Geometry: final body of the model. Coordinates: model frame, mm. A direction names the side the tool comes from. Coordinates: 2 decimals unless noted, no trailing zeros. Order: outer loops, then holes, each group sorted by start corner. A loop starts at its lowest first (then second) coordinate and runs counter-clockwise, first axis right, second up. Notation, with made-up numbers: (33.5, 85.5) - (87.5, 85.5) arc R20 cw to (87.5, 120.5) - close; hole circle Ø4 at (-2, 71.25). An arc over 180 degrees is marked (long way). Use one line per item in the form item = value. Start each with the question number.
```python
from build123d import *

# Parameters (mm, degrees)
CROQUIS1_R              = 1
CROQUIS1_R_2            = 1.25
SALIENTE_EXTRUIR1_DEPTH = 3
CORTAR_EXTRUIR1_DEPTH   = 1.5
CROQUIS3_R              = 2.1
CORTAR_EXTRUIR2_DEPTH   = 0.75
CROQUIS4_R              = 0.5
CORTAR_EXTRUIR3_DEPTH   = 23.410934831
CHAFL_N1_SIZE           = 0.5


with BuildPart() as part:
    # Croquis1 → Saliente-Extruir1 (new body)
    with BuildSketch(Plane.XY):
        with BuildLine():
            Line((0.210526316, 3.994455992), (19.157894737, 2.995841994))
            ThreePointArc((19.157894737, 2.995841994), (22, 0), (19.157894737, -2.995841994))
            Line((19.157894737, -2.995841994), (0.210526316, -3.994455992))
            ThreePointArc((0.210526316, -3.994455992), (-4, 0), (0.210526316, 3.994455992))
        make_face()
        Circle(CROQUIS1_R, mode=Mode.SUBTRACT)
        with Locations((19, 0)):
            Circle(CROQUIS1_R_2, mode=Mode.SUBTRACT)
    extrude(amount=SALIENTE_EXTRUIR1_DEPTH)

    # Croquis2 → Cortar-Extruir1 (cut)
    with BuildSketch(Plane(origin=(0, 0, 0), x_dir=(-1, 0, 0), z_dir=(0, 0, -1))):
        with BuildLine():
            Line((-15.154651163, 2.247564934), (-0.137209302, 2.946807358))
            ThreePointArc((-0.137209302, 2.946807358), (2.95, 0), (-0.137209302, -2.946807358))
            Line((-0.137209302, -2.946807358), (-15.154651163, -2.247564934))
            ThreePointArc((-15.154651163, -2.247564934), (-17.3, 0), (-15.154651163, 2.247564934))
        make_face()
    extrude(amount=-CORTAR_EXTRUIR1_DEPTH, mode=Mode.SUBTRACT)

    # Croquis3 → Cortar-Extruir2 (cut)
    with BuildSketch(Plane(origin=(0, 0, 1.5), x_dir=(-1, 0, 0), z_dir=(0, 0, -1))):
        Circle(CROQUIS3_R)
    extrude(amount=-CORTAR_EXTRUIR2_DEPTH, mode=Mode.SUBTRACT)

    # Croquis4 → Cortar-Extruir3 (cut, through all)
    with BuildSketch(Plane(origin=(0, 0, 1.5), x_dir=(-1, 0, 0), z_dir=(0, 0, -1))):
        with Locations((-15.05, 0)):
            Circle(CROQUIS4_R)
    extrude(amount=-CORTAR_EXTRUIR3_DEPTH, mode=Mode.SUBTRACT)

    # Chaflán1
    chafl_n1_edges = [part.edges().sort_by_distance(p)[0] for p in [
        (22, 0, 3),
        (9.684210526, 3.495148993, 3),
        (-4, 0, 3),
        (9.684210526, -3.495148993, 3),
    ]]
    chamfer(chafl_n1_edges, length=CHAFL_N1_SIZE)


solid = part.part
```
(1) Set-up query: faces 1 (the flat face through (7.751, 2.592, 0.74)), 2 (the cylindrical face through (22, 0, 1)). Return all of +Z, -Z, +X, -X, +Y, -Y with unobstructed straight access to the full face (end or side cutting, diameter ignored); none if empty.
(2) Cut plane A-A on y = 0. Return the cut outline in (x, z).
(3) Draft query along X for faces 3 (the cylindrical face through (14.573, 0.15, 2.24)), 4 (the flat face through (9.817, -3.488, 1.232)), 5 (the flat face through (9, 0, 3)). Return one class per face: released by +X, released by -X, zero draft, split by the parting line, or undercut.
(4) Contact query for flat-ended pins moving along their axis: pin 1 Ø2 at (x, y) = (19, 0) entering from +Z; pin 2 Ø1.5 at (x, y) = (10.5, -0.5) entering from -Z. Output: stop coordinate, or through.
(5) Cut plane C-C on x = 11.5. Return the cut outline in (y, z), plus the area to 3 significant figures.
(6) Material intervals for L1, parallel to X at y = -0.5, z = 0.7; L2, parallel to Z at x = 16, y = -0.25; L3, parallel to X at y = -1, z = 2.2, sorted ascending. Write a range as from..to.
(7) Cut plane D-D on x = 8.25. Return the cut outline in (y, z), plus the area to 3 significant figures.
Check sheet entries:
q1.face_1 = -Z
q1.face_2 = +Z, -Z, +X
q2.outline = (-4, 0) - (-2.95, 0) - (-2.95, 1.5) - (-2.1, 1.5) - (-2.1, 2.25) - (-1, 2.25) - (-1, 3) - (-3.5, 3) - (-4, 2.5) - close; (1, 2.25) - (2.1, 2.25) - (2.1, 1.5) - (14.55, 1.5) - (14.55, 3) - (1, 3) - close; (15.55, 1.5) - (17.3, 1.5) - (17.3, 0) - (17.75, 0) - (17.75, 3) - (15.55, 3) - close; (20.25, 0) - (22, 0) - (22, 2.5) - (21.5, 3) - (20.25, 3) - close
q3.face_3 = undercut
q3.face_4 = released by +X
q3.face_5 = zero draft
q4.pin_1 = through
q4.pin_2 = 1.5
q5.outline = (-3.4, 0) - (-2.42, 0) - (-2.42, 1.5) - (2.42, 1.5) - (2.42, 0) - (3.4, 0) - (3.4, 2.5) - (2.9, 3) - (-2.9, 3) - (-3.4, 2.5) - close
q5.area = 12.9 mm^2
q6.L1 = -3.97..-2.91, 17.24..17.85, 20.15..21.96
q6.L2 = 1.5..3
q6.L3 = -3.87..-1.85, 1.85..18.25, 19.75..21.83
q7.outline = (-3.57, 0) - (-2.57, 0) - (-2.57, 1.5) - (2.57, 1.5) - (2.57, 0) - (3.57, 0) - (3.57, 2.5) - (3.07, 3) - (-3.07, 3) - (-3.57, 2.5) - close
q7.area = 13.5 mm^2
